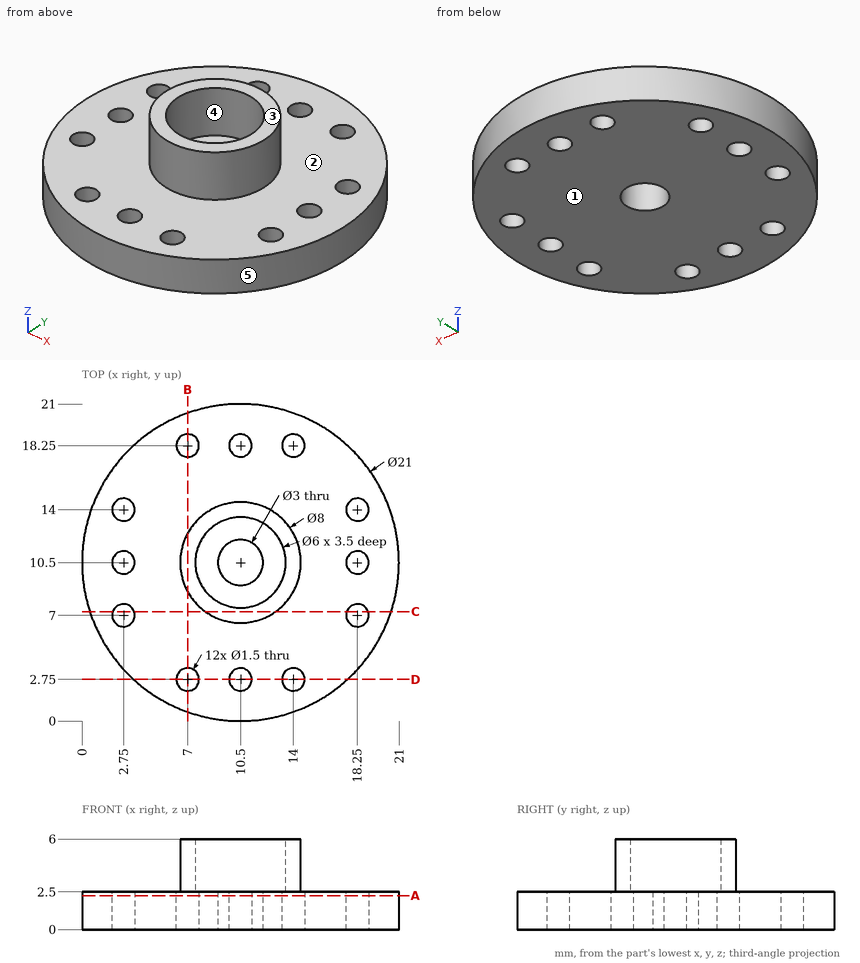
Can you work these out from the drawing? Everything is in mm from the part's minimum corner. A direction names the side the tool comes from. Round coordinates to 2 decimals unless told otherwise and drop trailing zeros. Order: outer loops, then holes, each group sorted by start corner. A loop starts at its lowest first (then second) coordinate and runs counter-clockwise, first axis right, second up. Notation, with made-up numbers: (-30.5, 49.5) -> (-17.5, 49.5) arc R24 cw to (-17.5, 83.5) -> close; hole circle Ø3 at (-9.75, -4). An arc over 180 degrees is marked (long way). Return JSON: item names as keys, results as strings. Group by question number.
1. If we section it at D-D, the plane y = 2.75: Write out the boundary of the cut face in (x, z), then the cut area to 3 significant figures.
2. If we section it at B-B, the plane x = 7: Write out the boundary of the cut face in (y, z).
3. I need wall thicknesses on line 1 (Y direction, x = 10.5, z = 0.9); line 2 (Y direction, x = 14, z = 1.35); line 3 (X direction, y = 2.5, z = 0.5). Which ranges of each line are inside material? Lowest first, please. Write a range as [from, to].
4. Will these pins go through, and if not, where does the flat tip stop? pin 1 (1.4 mm diameter, centred on x = 18.25, y = 14, fed in from -Z); pin 2 (1.5 mm diameter, centred on x = 14, z = 1, fed in from -Y); pin 3 (2 mm diameter, centred on x = 10.5, y = 2.75, fed in from -Z); pin 4 (1 mm diameter, centred on y = 15, z = 2.5, fed in from -X).
5. If we section it at A-A, the plane z = 2.25: Count the separate pieces of the cut face and the enclosed holes in it, then the cut area to 3 significant figures.
6. If we section it at C-C, the plane y = 7.25: Write out the boundary of the cut face in (x, z), then the cut area to 3 significant figures.
7. We'd pull the mould along X, two halves only. Please class the marked faces 3, 4 and 5: released by +X, released by -X, zero draft, split by the parting line, or undercut.
8. Which directions (+Z, -Z, +X, -X, +Y, -Y) give clear straight access to the entire face, cutting with the end or side of a thin tool? Please do the marked faces 1 and 2.
Output values:
{
 "1": {"outline": "(3.42, 0) -> (6.25, 0) -> (6.25, 2.5) -> (3.42, 2.5) -> close; (7.75, 0) -> (9.75, 0) -> (9.75, 2.5) -> (7.75, 2.5) -> close; (11.25, 0) -> (13.25, 0) -> (13.25, 2.5) -> (11.25, 2.5) -> close; (14.75, 0) -> (17.58, 0) -> (17.58, 2.5) -> (14.75, 2.5) -> close", "area": "24.2 mm²"},
 "2": {"outline": "(0.6, 0) -> (2, 0) -> (2, 2.5) -> (0.6, 2.5) -> close; (3.5, 0) -> (17.5, 0) -> (17.5, 2.5) -> (12.44, 2.5) -> (12.44, 6) -> (8.56, 6) -> (8.56, 2.5) -> (3.5, 2.5) -> close; (19, 0) -> (20.4, 0) -> (20.4, 2.5) -> (19, 2.5) -> close"},
 "3": {"line 1": "[0, 2], [3.5, 9], [12, 17.5], [19, 21]", "line 2": "[0.6, 2], [3.5, 17.5], [19, 20.4]", "line 3": "[3.7, 6.29], [7.71, 9.79], [11.21, 13.29], [14.71, 17.3]"},
 "4": {"pin 1": "through", "pin 2": "y = 0.37", "pin 3": "z = 0", "pin 4": "x = 0.79"},
 "5": {"separate pieces": "1", "enclosed holes": "13", "area": "318 mm²"},
 "6": {"outline": "(0.52, 0) -> (2.04, 0) -> (2.04, 2.5) -> (0.52, 2.5) -> close; (3.46, 0) -> (17.54, 0) -> (17.54, 2.5) -> (12.83, 2.5) -> (12.83, 6) -> (8.17, 6) -> (8.17, 2.5) -> (3.46, 2.5) -> close; (18.96, 0) -> (20.48, 0) -> (20.48, 2.5) -> (18.96, 2.5) -> close", "area": "59.2 mm²"},
 "7": {"face 3": "zero draft", "face 4": "undercut", "face 5": "split by the parting line"},
 "8": {"face 1": "-Z, +X, -X, +Y, -Y", "face 2": "+Z"}
}
